Autodesk Inventor part; units mm, degrees
ref_plane "YZ Plane" through (0, 0, 0) normal (1, 0, 0) x (0, 1, 0)
ref_plane "XZ Plane" through (0, 0, 0) normal (0, 1, 0) x (-1, 0, 0)
ref_plane "XY Plane" through (0, 0, 0) normal (0, 0, 1) x (1, 0, 0)
sketch "Sketch1" plane through (0, 0, 0) normal (0, 0, 1) x (1, 0, 0)
  line L0 (-9.525, -38.1) -> (9.525, -38.1)
  line L1 (9.525, -38.1) -> (9.525, 38.1)
  line L2 (9.525, 38.1) -> (-9.525, 38.1)
  line L3 (-9.525, 38.1) -> (-9.525, -38.1)
  line L4 (-9.525, -38.1) -> (9.525, 38.1) construction
  line L5 (9.525, -38.1) -> (-9.525, 38.1) construction
  line L6 (9.525, 38.1) -> (-9.525, 57.15)
  line L7 (-9.525, 57.15) -> (-9.525, 38.1)
  line L8 (-9.525, -38.1) -> (-9.525, -57.15)
  line L9 (-9.525, -57.15) -> (9.525, -38.1)
  point P0 (0, 0)
  dimension "d0" = 19.05
  dimension "d1" = 45
  dimension "d2" = 45
  dimension "d10" = 114.3
extrude "Extrusion1" add sketch "Sketch1" along normal mid plane 38.1
sketch "Sketch2" plane through (0, 0, 0) normal (0, 1, 0) x (-1, 0, 0)
  line L0 (6.35, 15.875) -> (-6.35, 15.875)
  line L1 (-6.35, 15.875) -> (-6.35, -15.875)
  line L2 (-6.35, -15.875) -> (6.35, -15.875)
  line L3 (6.35, -15.875) -> (6.35, 15.875)
  line L4 (6.35, 15.875) -> (-6.35, -15.875) construction
  line L5 (-6.35, 15.875) -> (6.35, -15.875) construction
  line L6 (-9.525, -19.05) -> (-9.525, 19.05)
  line L7 (-9.525, -19.05) -> (9.525, -19.05)
  point P0 (0, 0)
  dimension "d6" = 3.175
  dimension "d7" = 3.175
extrude "Extrusion2" cut sketch "Sketch2" along normal through all both and the other way through all
equation "\"d0\" = width"
equation "\"d10\" = length"
equation "\"d3\" = longSide"
equation "\"d8\" = longSide"
equation "\"width\" = 19.05"
equation "\"longSide\" = 38.1"
equation "\"length\" = 114.3"
properties part number "45dege0_75x1.50ForBottomOfShooter" material "Aluminum 6061"
Input: part model. Units: mm. Frame: model coordinates. A direction names the side the tool comes from. Round coordinates to 2 decimals unless told otherwise and drop trailing zeros. Loops run counter-clockwise (first coordinate to the right, second up) from the corner with the lowest first, then second, coordinate; pieces in that order, holes last. Notation, with made-up numbers: (61, 46) -> (77, 46) arc R13 ccw to (77, 50) -> close; hole circle Ø1 at (15, -25.75). An arc over 180 degrees is marked (long way). Answer as a JSON object with one key per item and string values. Group by question number.
1) Ray query, L1, parallel to Z at x = -3.5, y = -38 (3 decimals); L2, parallel to X at y = -27, z = 0.5 (3 decimals); L3, parallel to X at y = -43.5, z = 10 (3 decimals). Return the intervals inside material, ascending.
2) Section query B-B on y = -36.5. Output: boundary loops of the cut face in (x, z) (3 decimals).
3) Reachability of faces 5 (the flat face through (-9.525, 1, 0)), 6 (the flat face through (6.35, -1, 0)) from +Z, -Z, +X, -X, +Y, -Y: full face, straight path, thin tool, end or side. Return the list, or none.
4) Draft query along Z for faces 1 (the flat face through (0, 1, 19.05)), 2 (the flat face through (9.525, -1, 0)), 3 (the flat face through (0, -1, -15.875)), 4 (the flat face through (-6.35, -1, 0)). Return one class per face: +Z half, -Z half, draft (parallel to the pull), parting line (faces both ways), or undercut.
5) Section query A-A on z = 6. Output: boundary loops of the cut face in (x, y) (3 decimals).
6) Section query C-C on x = 3.75. Output: boundary loops of the cut face in (y, z) (3 decimals).
Reply:
{
 "1": {"L1": "z = -19.05 to -15.875, 15.875 to 19.05", "L2": "x = -9.525 to -6.35, 6.35 to 9.525", "L3": "x = -9.525 to -6.35"},
 "2": {"outline": "(-9.525, -19.05) -> (9.525, -19.05) -> (9.525, 19.05) -> (-9.525, 19.05) -> close; hole (-6.35, -15.875) -> (6.35, -15.875) -> (6.35, 15.875) -> (-6.35, 15.875) -> close"},
 "3": {"face 5": "+Z, -Z, -X, +Y, -Y", "face 6": "+Y, -Y"},
 "4": {"face 1": "+Z half", "face 2": "draft", "face 3": "undercut", "face 4": "undercut"},
 "5": {"outline": "(-9.525, -57.15) -> (-6.35, -53.975) -> (-6.35, 53.975) -> (-9.525, 57.15) -> close; (6.35, -41.275) -> (9.525, -38.1) -> (9.525, 38.1) -> (6.35, 41.275) -> close"},
 "6": {"outline": "(-43.875, -19.05) -> (43.875, -19.05) -> (43.875, -15.875) -> (-43.875, -15.875) -> close; (-43.875, 15.875) -> (43.875, 15.875) -> (43.875, 19.05) -> (-43.875, 19.05) -> close"}
}
